Check sheet for the modelled part. Datum: model origin and axes. Units: mm. Give positions to 0.01 mm unless a question says otherwise; leave off trailing zeros. Order: outer loops, then holes, each group sorted by start corner. A loop starts at its lowest first (then second) coordinate and runs counter-clockwise, first axis right, second up.
```python
from build123d import *

# Parameters (mm, degrees)
F0_W     = 25
F0_H     = 25
F1_DEPTH = 10
F3_DEPTH = 3
F3_TAPER = -20
F4_R     = 0.3


with BuildPart() as f1:
    # F0 (on Top) → F1 (new body)
    with BuildSketch(Plane.XY):
        Rectangle(F0_W, F0_H)
    extrude(amount=F1_DEPTH)

    # F2 (on face) → F3 (cut)
    with BuildSketch(Plane.YZ.offset(12.5)):
        Polygon((2.5, 10), (-2.5, 10), (-0.5, 0), (0.5, 0), align=None)
    extrude(amount=-F3_DEPTH, taper=F3_TAPER, mode=Mode.SUBTRACT)

    # F4
    f4_edges = [f1.edges().sort_by_distance(p)[0] for p in [
        (-12.5, 0, 0),
        (0, 12.5, 0),
        (12.5, 6.5, 0),
        (11, 1.056767, 0),
        (9.5, 0, 0),
        (11, -1.056767, 0),
        (12.5, -6.5, 0),
        (0, -12.5, 0),
    ]]
    fillet(f4_edges, radius=F4_R)


solid = f1.part
```
(1) Release check for a two-part mould opening along X. For faces 1 (the face through (9.5, 0, 6)), 2 (the face through (0, 12.5, 5)), 3 (the face through (-12.5, 0, 5)) record: released by +X, released by -X, zero draft, split by the parting line, or undercut.
Response values:
face 1: undercut
face 2: zero draft
face 3: released by -X
(2) Material ranges on L1, parallel to Y at x = 11, z = 8, recorded low to high.
Response values:
L1: y = -12.5 to -2.66, 2.66 to 12.5
(3) Cross-section at A-A on y = 0.25. Enter the section's corners in (x, z), then the cut area to 3 significant figures.
Response values:
outline: (-12.5, 0.3) arc R0.3 ccw to (-12.2, 0) - (9.2, 0) arc R0.3 ccw to (9.5, 0.3) - (9.5, 10) - (-12.5, 10) - close
area: 220 mm2
